Here's the drawing with two shaded views (mm, measured from the low corner). I have some questions. A direction names the side the tool comes from. Coordinates: 2 decimals unless noted, no trailing zeros. Write each loop counter-clockwise with the first axis right and the second up, starting at its lowest first coordinate (ties: lowest second). Pieces come first, ordered by that corner, then holes. Notation, with made-up numbers: (0.25, 68) - (5.25, 68) arc R13 cw to (5.25, 80) - close; hole circle Ø9 at (-12, -29.75). An arc over 180 degrees is marked (long way). Answer in a Markdown table with one row per item. Add a question column.
Item 1: Imagine slicing it at D-D (y = 21.5). Please give me the cut outline in (x, z), plus the area to 3 significant figures.
Item 2: Imagine slicing it at A-A (y = 2). Please give me the cut outline in (x, z), plus the area to 3 significant figures.
Item 3: We'd pull the mould along X, two halves only. Please class the marked faces 4, 5 and 6: +X half, -X half, draft (parallel to the pull), parting line (faces both ways), or undercut.
Item 4: If I drill on probe 1 along X at (y, z) = (1.3, 5); probe 2 along Y at (x, z) = (8.75, 7); probe 3 along X at (y, z) = (26.5, 1.75), over which ranges is the centre line in solid material (lowest first)? Write a range as from..to.
Item 5: Imagine slicing it at C-C (y = 24.75). Please give me the cut outline in (x, z), plus the area to 3 significant figures.
Item 6: Imagine slicing it at B-B (z = 1). Please give me the cut outline in (x, y).
Item 7: Which directions (+Z, -Z, +X, -X, +Y, -Y) give clear straight access to the entire face, cutting with the end or side of a thin tool? Please do the marked faces 1, 2 and 3.
Item 8: I'm going to push flat-ended pins straight in: pin 1 (3 mm diameter, centred on x = 23, y = 4.5, fed in from +Z); pin 2 (3 mm diameter, centred on x = 5, z = 5, fed in from +Y); pin 3 (4.5 mm diameter, centred on x = 21, z = 7, fed in from +Y); pin 4 (1 mm diameter, centred on y = 6.5, z = 2.5, fed in from -X). Where does each tip first touch, or does it pass through?
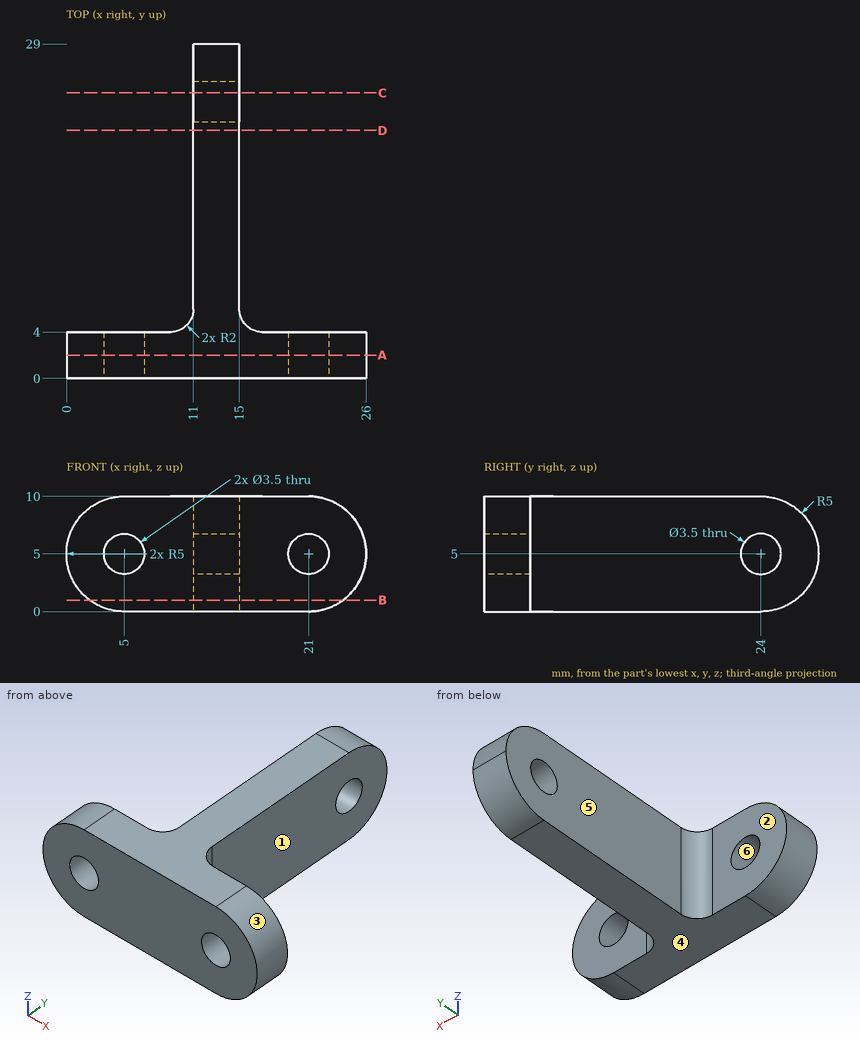
Here are the results:
| question | item | result |
|---|---|---|
| 1 | outline | (11, 0) - (15, 0) - (15, 10) - (11, 10) - close |
| 1 | area | 40.0 mm2 |
| 2 | outline | (5, 0) - (21, 0) arc R5 ccw to (21, 10) - (5, 10) arc R5 ccw to start; hole circle Ø3.5 at (5, 5); hole circle Ø3.5 at (21, 5) |
| 2 | area | 219 mm2 |
| 3 | face 4 | draft |
| 3 | face 5 | -X half |
| 3 | face 6 | undercut |
| 4 | probe 1 | x = 0..3.25, 6.75..19.25, 22.75..26 |
| 4 | probe 2 | y = 0..4 |
| 4 | probe 3 | x = 11..15 |
| 5 | outline | (11, 0.06) - (15, 0.06) - (15, 3.42) - (11, 3.42) - close; (11, 6.58) - (15, 6.58) - (15, 9.94) - (11, 9.94) - close |
| 5 | area | 26.9 mm2 |
| 6 | outline | (2, 0) - (24, 0) - (24, 4) - (17, 4) arc R2 cw to (15, 6) - (15, 27) - (11, 27) - (11, 6) arc R2 cw to (9, 4) - (2, 4) - close |
| 7 | face 1 | +Z, -Z, +X, +Y |
| 7 | face 2 | +Z, -Z, -X, +Y |
| 7 | face 3 | +X, +Y, -Y |
| 8 | pin 1 | stops at z = 9.97 |
| 8 | pin 2 | passes through |
| 8 | pin 3 | stops at y = 4 |
| 8 | pin 4 | stops at x = 11 |
